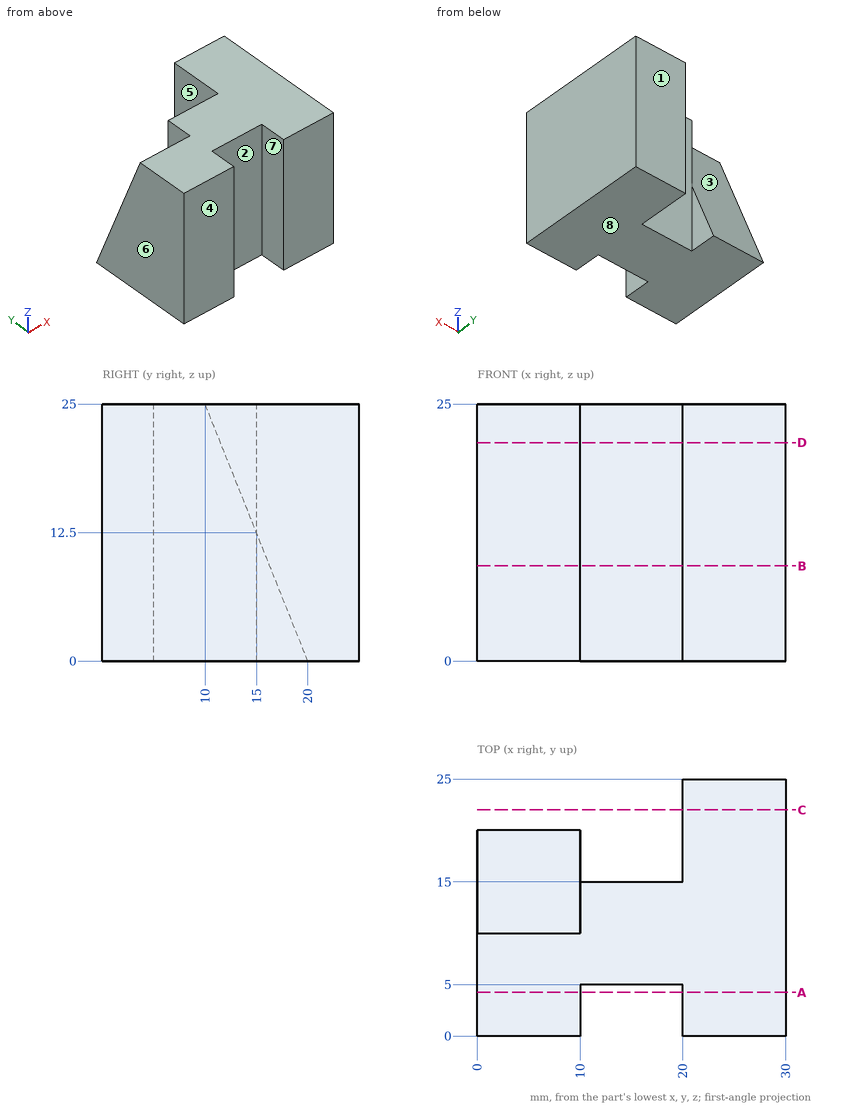
Can you work these out from the drawing? Everything is in mm from the part's minimum corner. A direction names the side the tool comes from. Coordinates: 2 decimals unless noted, no trailing zeros. Write each loop counter-clockwise with the first axis right and the second up, starting at its lowest first coordinate (ties: lowest second). Pieces come first, ordered by that corner, then holes. Notation, with made-up numbers: (67.5, -9) - (114.5, -9) arc R18 ccw to (114.5, 15) - close; hole circle Ø11 at (2, 18). An arc over 180 degrees is marked (long way). One line per item, written item: value.
1) I'm going to push flat-ended pins straight in: P1, Ø5, axis at x = 13, z = 16, coming from the -Y side; P2, Ø8, axis at x = 13, z = 18, coming from the +Y side. Where does each tip first touch, or does it pass through?
Model answer:
P1: stops at y = 5
P2: stops at y = 15
2) Suppose I cut it at A-A on y = 4.25. Write out the boundary of the cut face in (x, z), and give its area (3 significant figures).
Model answer:
outline: (0, 0) - (10, 0) - (10, 25) - (0, 25) - close; (20, 0) - (30, 0) - (30, 25) - (20, 25) - close
area: 500 mm²
3) Suppose I cut it at C-C on y = 22. Write out the boundary of the cut face in (x, z).
Model answer:
outline: (20, 0) - (30, 0) - (30, 25) - (20, 25) - close
4) We'd pull the mould along X, two halves only. Please class the marked faces 6, 7 and 8: pulls with the +X half, pulls with the -X half, needs draft (parallel to the pull), parting line crosses it, or undercut.
Model answer:
face 6: pulls with the -X half
face 7: undercut
face 8: needs draft
5) I need wall thicknesses on line 1 along X through (y, z) = (3, 19.25); line 2 along Y through (x, z) = (11.75, 23.25); line 3 along X through (y, z) = (23, 13.5). Which ranges of each line are inside material? Lowest first, please.
Model answer:
line 1: x = 0 to 10, 20 to 30
line 2: y = 5 to 15
line 3: x = 20 to 30
6) Suppose I cut it at B-B on z = 9.25. Write out the boundary of the cut face in (x, y), and give its area (3 significant figures).
Model answer:
outline: (0, 0) - (10, 0) - (10, 5) - (20, 5) - (20, 0) - (30, 0) - (30, 25) - (20, 25) - (20, 15) - (10, 15) - (10, 16.3) - (0, 16.3) - close
area: 513 mm²
7) On a 3-axis mill with a long thin cutter (end or side, diameter ignored), from which of +Z, -Z, +X, -X, +Y, -Y can I reach the whole of each face in a straight line? I mean the marked faces 1, 2, 3, 4 and 5. Say none if no direction works.
Model answer:
face 1: +Z, -Z, +X, -X, +Y
face 2: +Z, -Z, -Y
face 3: +Z, -X, +Y
face 4: +Z, -Z, +X, -X, -Y
face 5: +Z, -Z, +Y
8) Suppose I cut it at D-D on z = 21.25. Write out the boundary of the cut face in (x, y), and give its area (3 significant figures).
Model answer:
outline: (0, 0) - (10, 0) - (10, 5) - (20, 5) - (20, 0) - (30, 0) - (30, 25) - (20, 25) - (20, 15) - (10, 15) - (10, 11.5) - (0, 11.5) - close
area: 465 mm²
